from build123d import *

# Parameters (mm, degrees)
F0_W = 1.5
F0_H = 3.25


with BuildPart() as f1:
    # F0 (on Front) → F1 (revolve)
    with BuildSketch(Plane.XZ):
        with BuildLine():
            Line((-9.269153, 7.75), (-9.269153, 11))
            Line((-9.269153, 11), (-10.758264, 10.144415))
            ThreePointArc((-10.758264, 10.144415), (-11.392868, 9.724113), (-11.969153, 9.226848))
            ThreePointArc((-11.969153, 9.226848), (-12.191108, 8.900003), (-12.269153, 8.512705))
            Line((-12.269153, 8.512705), (-12.269153, 7.75))
            Line((-12.269153, 7.75), (-9.269153, 7.75))
        make_face()
        with Locations((-8.519153, 9.375)):
            Rectangle(F0_W, F0_H)
    revolve(axis=Axis((-10.019153, 0, 5.5), (1, 0, 0)))


solid = f1.part
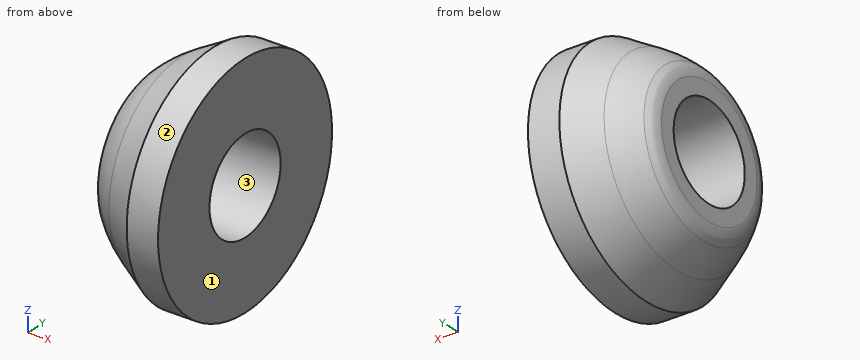
Read the model definition and answer for the solid it produces. Units are mm, in the model's axes. Face numbers are marked on the shaded views. Round coordinates to 2 decimals unless told otherwise and drop trailing zeros. Write each loop counter-clockwise with the first axis right and the second up, starting at its lowest first coordinate (ties: lowest second). Pieces come first, ordered by that corner, then holes.
1. Given pin 1 Ø2 at (x, y) = (-11.5, -1) entering from -Z; pin 2 Ø1.5 at (x, y) = (-11, -1.5) entering from +Z, each flat-ended and moving along its own axis, determine where each tip first touches the part or whether it passes through.
2. The part is cut by section B-B, the plane x = -10.4. Determine the outline of the cut face in (y, z).
3. Determine the mould class of the marked faces 1, 2 and 3 for opening direction Z: pulls with the +Z half, pulls with the -Z half, needs draft (parallel to the pull), parting line crosses it, or undercut.
4. The part is cut by section A-A, the plane x = -8.15. Determine the outline of the cut face in (y, z), then the cut area to 3 significant figures.
5. Straight lines are drawn through the part: L1, parallel to Y at x = -10.2, z = 5.5; L2, parallel to Z at x = -8.75, y = 0; L3, parallel to Y at x = -11.4, z = 4.25. For each, find the intervals that lie inside material, in ascending order.
Values:
1. pin 1: stops at z = 0.78
1. pin 2: stops at z = 10.25
2. outline: circle Ø9.7 at (0, 5.5); hole circle Ø4.5 at (0, 5.5)
3. face 1: needs draft
3. face 2: parting line crosses it
3. face 3: undercut
4. outline: circle Ø11 at (0, 5.5); hole circle Ø4.5 at (0, 5.5)
4. area: 79.1 mm2
5. L1: y = -4.97 to -2.25, 2.25 to 4.97
5. L2: z = 0 to 3.25, 7.75 to 11
5. L3: y = -4.03 to -1.87, 1.87 to 4.03
